from build123d import *
from build123d.topology import SkipClean

# Parameters (mm, degrees)
SKETCH2_R           = 85
SKETCH2_R_2         = 20
BOSS_EXTRUDE1_DEPTH = 5
BOSS_EXTRUDE2_START = 155
SKETCH3_W           = 245
SKETCH3_H           = 230
SKETCH3_R           = 85
SKETCH3_W_2         = 265
SKETCH3_H_2         = 285
SKETCH3_R_2         = 20
BOSS_EXTRUDE2_DEPTH = 155
SKETCH4_W           = 33
SKETCH4_H           = 40
BOSS_EXTRUDE4_DEPTH = 70
SKETCH6_R           = 15
SKETCH6_W           = 63
SKETCH6_H           = 50
BOSS_EXTRUDE6_DEPTH = 22
SKETCH6_3_R         = 15
SKETCH6_3_R_2       = 6
BOSS_EXTRUDE7_DEPTH = 47
SKETCH6_4_R         = 6
BOSS_EXTRUDE8_DEPTH = 77


with BuildPart() as part:
    # Sketch2 → Boss-Extrude1 (new body)
    with BuildSketch(Plane.XY):
        Circle(SKETCH2_R)
        Circle(SKETCH2_R_2, mode=Mode.SUBTRACT)
    extrude(amount=BOSS_EXTRUDE1_DEPTH)

    # Sketch3 → Boss-Extrude2 (add)
    # profile 1 of 3: a face of its own
    with SkipClean():  # the faces are left unmerged after this step: merging them gives an invalid solid
        with BuildSketch(Plane(origin=(0, 0, 0), x_dir=(-1, 0, 0), z_dir=(0, 0, -1)).offset(BOSS_EXTRUDE2_START)):
            with Locations((-17.5, -20)):
                Rectangle(SKETCH3_W, SKETCH3_H)
            with Locations(Location((0, 0, 0), (0, 0, 180))):
                Circle(SKETCH3_R, mode=Mode.SUBTRACT)
        # profile 2 of 3: a face of its own
        with BuildSketch(Plane(origin=(0, 0, 0), x_dir=(-1, 0, 0), z_dir=(0, 0, -1)).offset(BOSS_EXTRUDE2_START)):
            with Locations((-272.5, 7.5)):
                Rectangle(SKETCH3_W_2, SKETCH3_H_2)
        # profile 3 of 3: a face of its own
        with BuildSketch(Plane(origin=(0, 0, 0), x_dir=(-1, 0, 0), z_dir=(0, 0, -1)).offset(BOSS_EXTRUDE2_START)):
            with Locations(Location((0, 0, 0), (0, 0, 180))):
                Circle(SKETCH3_R)
            Circle(SKETCH3_R_2, mode=Mode.SUBTRACT)
        extrude(amount=-BOSS_EXTRUDE2_DEPTH)

    # Sketch4 → Boss-Extrude4 (add)
    with SkipClean():  # the faces are left unmerged after this step: merging them gives an invalid solid
        with BuildSketch(Plane(origin=(0, 0, -155), x_dir=(-1, 0, 0), z_dir=(0, 0, -1))):
            with Locations((-83.5, 115)):
                Rectangle(SKETCH4_W, SKETCH4_H)
        extrude(amount=-BOSS_EXTRUDE4_DEPTH)

    # Sketch6 → Boss-Extrude6 (add)
    # profile 1 of 2: a face of its own
    with SkipClean():  # the faces are left unmerged after this step: merging them gives an invalid solid
        with BuildSketch(Plane.XZ.offset(135)):
            Polygon((-115, 50), (-115, 0), (-105, 0), (-52, 0), (-52, 50), align=None)
            with Locations(Location((-83.5, 25, 0), (0, 0, 270))):
                Circle(SKETCH6_R, mode=Mode.SUBTRACT)
        # profile 2 of 2: a face of its own
        with BuildSketch(Plane.XZ.offset(135)):
            with Locations((83.5, 25)):
                Rectangle(SKETCH6_W, SKETCH6_H)
            with Locations(Location((83.5, 25, 0), (0, 0, 270))):
                Circle(SKETCH6_R, mode=Mode.SUBTRACT)
        extrude(amount=-BOSS_EXTRUDE6_DEPTH)

    # Sketch6_3 → Boss-Extrude7 (add)
    # profile 1 of 2: a face of its own
    with SkipClean():  # the faces are left unmerged after this step: merging them gives an invalid solid
        with BuildSketch(Plane.XZ.offset(135)):
            with Locations(Location((-83.5, 25, 0), (0, 0, 270))):
                Circle(SKETCH6_3_R)
            with Locations(Location((-83.5, 25, 0), (0, 0, 270))):
                Circle(SKETCH6_3_R_2, mode=Mode.SUBTRACT)
        # profile 2 of 2: a face of its own
        with BuildSketch(Plane.XZ.offset(135)):
            with Locations(Location((83.5, 25, 0), (0, 0, 270))):
                Circle(SKETCH6_3_R)
            with Locations(Location((83.5, 25, 0), (0, 0, 270))):
                Circle(SKETCH6_3_R_2, mode=Mode.SUBTRACT)
        extrude(amount=-BOSS_EXTRUDE7_DEPTH)

    # Sketch6_4 → Boss-Extrude8 (add)
    with SkipClean():  # the faces are left unmerged after this step: merging them gives an invalid solid
        with BuildSketch(Plane.XZ.offset(135)):
            with Locations(Location((-83.5, 25, 0), (0, 0, 270))):
                Circle(SKETCH6_4_R)
            with Locations(Location((83.5, 25, 0), (0, 0, 270))):
                Circle(SKETCH6_4_R)
        extrude(amount=-BOSS_EXTRUDE8_DEPTH)


solid = part.part
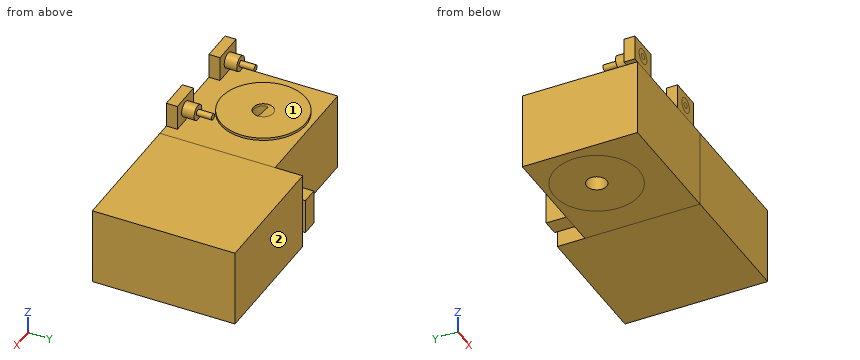
CAD build for the part. Positions are in the model's coordinates, mm. Face numbers are marked on the shaded views. A direction names the side the tool comes from. Coordinates: 2 decimals unless noted, no trailing zeros. Order: outer loops, then holes, each group sorted by start corner. A loop starts at its lowest first (then second) coordinate and runs counter-clockwise, first axis right, second up.
Item 1: Band-saw the part on A-A on y = -102. List the corners of the cut face in (x, z), plus the area to 3 significant figures.
Check sheet entries:
outline: (-105, -155) - (405, -155) - (405, 0) - (-105, 0) - close; circle Ø30 at (-83.5, 25); circle Ø30 at (83.5, 25)
area: 80,500 mm2
Item 2: 3-axis set-ups, long thin cutter, end or side, ignore diameter. For the marked faces 1 and 2: which of +Z, -Z, +X, -X, +Y, -Y reach the whole face in a straight line?
Check sheet entries:
face 1: +Z, +X, -X, +Y
face 2: +Z, -Z, +X, -X, +Y
Item 3: Drill centre lines: L1, parallel to Y at x = 0, z = -113; L2, parallel to X at y = 97, z = -91; L3, parallel to X at y = 0, z = -74. Where is each one in solid material? Low to high.
Check sheet entries:
L1: y = -135 to -20, 20 to 95
L2: x = 67 to 100, 140 to 405
L3: x = -105 to -20, 20 to 405
Item 4: Band-saw the part on D-D on y = 40. List the corners of the cut face in (x, z).
Check sheet entries:
outline: (-105, -155) - (405, -155) - (405, 0) - (75, 0) - (75, 5) - (-75, 5) - (-75, 0) - (-105, 0) - close
Item 5: Band-saw the part on C-C on z = -127. List the corners of the cut face in (x, y), plus the area to 3 significant figures.
Check sheet entries:
outline: (-105, -135) - (405, -135) - (405, 150) - (140, 150) - (140, 95) - (100, 95) - (100, 135) - (67, 135) - (67, 95) - (-105, 95) - close; hole circle Ø40 at (0, 0)
area: 132,000 mm2
Item 6: Pin check, flat tips, straight feed: pin 1 Ø2 at (x, y) = (68, 90.5) entering from +Z; pin 2 Ø25 at (x, z) = (94, 22.5) entering from +Y; pin 3 Ø3 at (x, z) = (55, -9) entering from +Y; pin 4 Ø1.5 at (y, z) = (-69, 7) entering from +X. Stop position of each tip, or through.
Check sheet entries:
pin 1: stops at z = 0
pin 2: stops at y = -58
pin 3: stops at y = 95
pin 4: passes through
Item 7: Band-saw the part on B-B on z = 25. List the corners of the cut face in (x, y).
Check sheet entries:
outline: (-115, -135) - (-52, -135) - (-52, -113) - (-68.5, -113) - (-68.5, -88) - (-77.5, -88) - (-77.5, -58) - (-89.5, -58) - (-89.5, -88) - (-98.5, -88) - (-98.5, -113) - (-115, -113) - close; (52, -135) - (115, -135) - (115, -113) - (98.5, -113) - (98.5, -88) - (89.5, -88) - (89.5, -58) - (77.5, -58) - (77.5, -88) - (68.5, -88) - (68.5, -113) - (52, -113) - close
